Geometry: final body of the model. Coordinates: model frame, mm. Give positions to 0.01 mm unless a question says otherwise; leave off trailing zeros. Write each loop counter-clockwise with the first axis right and the second up, starting at its lowest first coordinate (ties: lowest second). Pieces come first, ordered by that corner, then holes.
from build123d import *

# Parameters (mm, degrees)
F0_W      = 127
F0_H      = 127
F1_DEPTH  = 127
F2_R      = 11.1125
F3_DEPTH  = 6.35
F4_R      = 11.1125
F5_DEPTH  = 6.35
F6_R      = 11.1125
F7_DEPTH  = 6.35
F8_R      = 11.1125
F9_DEPTH  = 6.35
F10_R     = 11.1125
F11_DEPTH = 6.35
F12_R     = 11.1125
F13_DEPTH = 6.35


with BuildPart() as f1:
    # F0 (on Top) → F1 (new body)
    with BuildSketch(Plane.XY):
        with Locations((63.5, -63.5)):
            Rectangle(F0_W, F0_H)
    extrude(amount=F1_DEPTH)

    # F2 (on face) → F3 (cut)
    with BuildSketch(Plane(origin=(0, 0, 0), x_dir=(1, 0, 0), z_dir=(0, 0, -1))):
        with Locations((63.5, 63.5)):
            Circle(F2_R)
    extrude(amount=-F3_DEPTH, mode=Mode.SUBTRACT)

    # F4 (on face) → F5 (cut)
    with BuildSketch(Plane(origin=(0, 0, 0), x_dir=(0, -1, 0), z_dir=(-1, 0, 0))):
        with Locations((99.731132, 104.775)):
            Circle(F4_R)
        with Locations((22.225, 22.225)):
            Circle(F4_R)
    extrude(amount=-F5_DEPTH, mode=Mode.SUBTRACT)

    # F6 (on face) → F7 (cut)
    with BuildSketch(Plane(origin=(0, 0, 0), x_dir=(-1, 0, 0), z_dir=(0, 1, 0))):
        with Locations((-22.225, 104.775)):
            Circle(F6_R)
        with Locations((-63.5, 63.5)):
            Circle(F6_R)
        with Locations((-104.775, 22.225)):
            Circle(F6_R)
    extrude(amount=-F7_DEPTH, mode=Mode.SUBTRACT)

    # F8 (on face) → F9 (cut)
    with BuildSketch(Plane.XY.offset(127)):
        with Locations((22.225, -22.225)):
            Circle(F8_R)
        with Locations((22.225, -60.325)):
            Circle(F8_R)
        with Locations((22.225, -104.775)):
            Circle(F8_R)
        with Locations((104.775, -60.325)):
            Circle(F8_R)
        with Locations((104.775, -104.775)):
            Circle(F8_R)
        with Locations((104.775, -22.225)):
            Circle(F8_R)
    extrude(amount=-F9_DEPTH, mode=Mode.SUBTRACT)

    # F10 (on face) → F11 (cut)
    with BuildSketch(Plane.XZ.offset(127)):
        with Locations((104.775, 22.225)):
            Circle(F10_R)
        with Locations((104.775, 104.775)):
            Circle(F10_R)
        with Locations((22.225, 104.775)):
            Circle(F10_R)
        with Locations((22.225, 22.225)):
            Circle(F10_R)
    extrude(amount=-F11_DEPTH, mode=Mode.SUBTRACT)

    # F12 (on face) → F13 (cut)
    with BuildSketch(Plane.YZ.offset(127)):
        with BuildLine():
            ThreePointArc((-11.1125, 104.775), (-11.958389, 109.02757), (-14.367276, 112.632724))
            Line((-14.367276, 112.632724), (-30.082724, 96.917276))
            ThreePointArc((-30.082724, 96.917276), (-17.97243, 94.508389), (-11.1125, 104.775))
        make_face()
        with BuildLine():
            ThreePointArc((-93.6625, 22.225), (-94.508389, 26.47757), (-96.917276, 30.082724))
            Line((-96.917276, 30.082724), (-112.632724, 14.367276))
            ThreePointArc((-112.632724, 14.367276), (-100.52243, 11.958389), (-93.6625, 22.225))
        make_face()
        with BuildLine():
            Line((-112.632724, 14.367276), (-96.917276, 30.082724))
            ThreePointArc((-96.917276, 30.082724), (-112.632724, 30.082724), (-112.632724, 14.367276))
        make_face()
        with BuildLine():
            ThreePointArc((-52.3875, 63.5), (-53.233389, 67.75257), (-55.642276, 71.357724))
            Line((-55.642276, 71.357724), (-71.357724, 55.642276))
            ThreePointArc((-71.357724, 55.642276), (-59.24743, 53.233389), (-52.3875, 63.5))
        make_face()
        with BuildLine():
            Line((-71.357724, 55.642276), (-55.642276, 71.357724))
            ThreePointArc((-55.642276, 71.357724), (-71.357724, 71.357724), (-71.357724, 55.642276))
        make_face()
        with BuildLine():
            Line((-30.082724, 96.917276), (-14.367276, 112.632724))
            ThreePointArc((-14.367276, 112.632724), (-30.082724, 112.632724), (-30.082724, 96.917276))
        make_face()
        with Locations((-22.225, 22.225)):
            Circle(F12_R)
        with Locations((-104.775, 104.775)):
            Circle(F12_R)
    extrude(amount=-F13_DEPTH, mode=Mode.SUBTRACT)


solid = f1.part
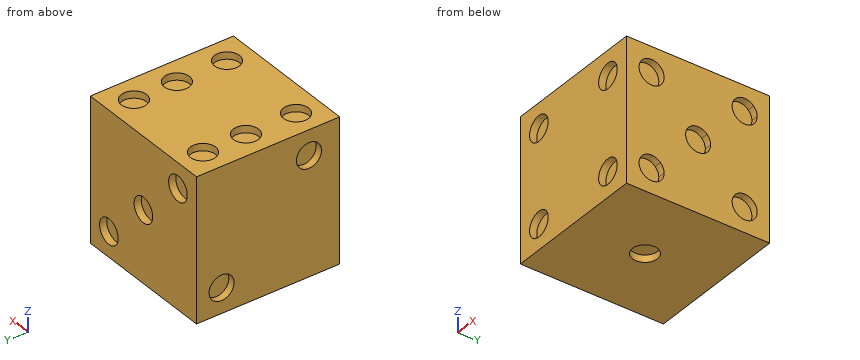
Q1. Section B-B on y = -99. Output: boundary loops of the cut face in (x, z).
Filled sheet:
outline: (0, 0) - (127, 0) - (127, 12.73) - (120.65, 12.73) - (120.65, 31.72) - (127, 31.72) - (127, 95.28) - (120.65, 95.28) - (120.65, 114.27) - (127, 114.27) - (127, 127) - (114.27, 127) - (114.27, 120.65) - (95.28, 120.65) - (95.28, 127) - (31.72, 127) - (31.72, 120.65) - (12.73, 120.65) - (12.73, 127) - (0, 127) - (0, 115.86) - (6.35, 115.86) - (6.35, 93.69) - (0, 93.69) - close
Q2. Section A-A on x = 63.5. Output: boundary loops of the cut face in (y, z), plus the area to 3 significant figures.
Filled sheet:
outline: (-127, 0) - (-74.61, 0) - (-74.61, 6.35) - (-52.39, 6.35) - (-52.39, 0) - (0, 0) - (0, 52.39) - (-6.35, 52.39) - (-6.35, 74.61) - (0, 74.61) - (0, 127) - (-127, 127) - close
area: 15,800 mm2
Q3. Pin query (flat end, axial travel): P1, Ø18, axis at x = 104.775, z = 22.225, coming from the -Y side; P2, Ø11, axis at x = 109, z = 23, coming from the +Y side. Return the tip coordinate at first contact, or that it passes through.
Filled sheet:
P1: stops at y = -120.65
P2: stops at y = -6.35
Q4. Ray query, line 1 along X through (y, z) = (-63.5, 1.5); line 2 along X through (y, z) = (-58.5, 121); line 3 along Y through (x, z) = (29, 110.5). Return the intervals inside material, ascending.
Filled sheet:
line 1: x = 0 to 52.39, 74.61 to 127
line 2: x = 0 to 11.26, 33.19 to 93.81, 115.74 to 127
line 3: y = -120.65 to -6.35
Q5. Section D-D on y = -63.5. Output: boundary loops of the cut face in (x, z), plus the area to 3 significant figures.
Filled sheet:
outline: (0, 0) - (52.39, 0) - (52.39, 6.35) - (74.61, 6.35) - (74.61, 0) - (127, 0) - (127, 52.39) - (120.65, 52.39) - (120.65, 74.61) - (127, 74.61) - (127, 127) - (115.42, 127) - (115.42, 120.65) - (94.13, 120.65) - (94.13, 127) - (32.87, 127) - (32.87, 120.65) - (11.58, 120.65) - (11.58, 127) - (0, 127) - close
area: 15,600 mm2
Q6. Section C-C on x = 28. Output: boundary loops of the cut face in (y, z), plus the area to 3 significant figures.
Filled sheet:
outline: (-127, 0) - (0, 0) - (0, 95.28) - (-6.35, 95.28) - (-6.35, 114.27) - (0, 114.27) - (0, 127) - (-12.73, 127) - (-12.73, 120.65) - (-31.72, 120.65) - (-31.72, 127) - (-50.83, 127) - (-50.83, 120.65) - (-69.82, 120.65) - (-69.82, 127) - (-95.28, 127) - (-95.28, 120.65) - (-114.27, 120.65) - (-114.27, 127) - (-127, 127) - (-127, 114.27) - (-120.65, 114.27) - (-120.65, 95.28) - (-127, 95.28) - (-127, 31.72) - (-120.65, 31.72) - (-120.65, 12.73) - (-127, 12.73) - close
area: 15,400 mm2
